CAD build for the part. Positions are in the model's coordinates, mm. A direction names the side the tool comes from. Give positions to 0.01 mm unless a question says otherwise; leave off trailing zeros. Write each loop counter-clockwise with the first axis right and the second up, starting at its lowest first coordinate (ties: lowest second). Pieces come first, ordered by that corner, then holes. Notation, with made-up numbers: (86, -18) - (116, -18) arc R29 cw to (116, 3) - close; hole circle Ø3 at (33, -35). An arc over 180 degrees is marked (long way). Answer as a JSON object with one key per item and string values.
Autodesk Inventor part; units mm, degrees
ref_plane "Work Plane1" through (1.525, 0, 0) normal (0, 0, 1) x (1, 0, 0)
ref_plane "YZ Plane" through (0, 0, 0) normal (1, 0, 0) x (0, 1, 0)
ref_plane "XZ Plane" through (0, 0, 0) normal (0, 1, 0) x (-1, 0, 0)
sketch "Sketch1" plane through (0, 0, 0) normal (0, 0, 1) x (1, 0, 0)
  line L0 (0, 3) -> (12, 3)
  line L1 (12, 3) -> (12, 0)
  line L2 (12, 0) -> (0, 0)
  line L3 (-2.4, 0) -> (14.4, 0)
  line L4 (0, -0.6) -> (0, 3.6)
  line L5 (0, 3) -> (0, 0)
  dimension "d2" = 6
  dimension "d59" = 12
revolve "Body" add sketch "Sketch1" angle 360 about axis through (12, 0, 0) along (-1, 0, 0)
sketch "Sketch2" plane through (0, 0, 0) normal (-1, 0, 0) x (0, 0, 1)
  line L0 (0, 5.7735) -> (5, 2.8868)
  line L1 (5, 2.8868) -> (5, -2.8868)
  line L2 (5, -2.8868) -> (0, -5.7735)
  line L3 (0, -5.7735) -> (-5, -2.8868)
  line L4 (-5, -2.8868) -> (-5, 2.8868)
  line L5 (-5, 2.8868) -> (0, 5.7735)
  line L6 (-7, 0) -> (7, 0)
  line L7 (0, 8.0829) -> (0, -8.0829)
  point P0 (0, 0)
  point P1 (0, 0)
  dimension "d11" = 10
extrude "Head" add sketch "Sketch2" along normal blind 4
sketch "Sketch4" plane through (0, 0, 0) normal (0, 0, 1) x (1, 0, 0)
  line L0 (-3.4226, 6) -> (-4, 5)
  line L1 (-1.1, 0) -> (-0.234, 0)
  line L2 (-4.7532, 0) -> (0.5192, 0)
  line L3 (-4, 6) -> (-3.4226, 6)
  line L4 (-4, 5) -> (-4, 6)
  line L5 (0, 7.2) -> (0, -1.2)
  dimension "d65" = 10
  dimension "d67" = 30
  dimension "d68" = 12
  dimension "d69" = 4
revolve "Chamfer1" cut sketch "Sketch4" angle 360 about axis through (-1.1, 0, 0) along (1, 0, 0)
thread "Thread"
chamfer "Chamfer2" distance 0.6135 distance2 0.6136 1 edges at (12, -3, 0) measured on face at (12, -0.8855, 0.4647)
fillet "Fillet2" radius 0.25 1 edges at (0, -3, 0)
ref_plane "Work Plane1" through (1.525, 0, 0) normal (0, 0, 1) x (1, 0, 0)
equation "\"d2\" = GD"
equation "\"d59\" = NLG"
equation "\"d11\" = SW"
equation "\"d3\" = KOH"
equation "\"d71\" = RR"
equation "\"d15\" = GEL"
equation "\"d6\" = -0.5 * SPD + 0.5 * GD"
equation "\"d65\" = SW"
equation "\"d67\" = ANG1"
equation "\"d68\" = 1.2 * SW"
equation "\"d69\" = KOH"
equation "\"NLG\" = 12"
equation "\"GD\" = NND"
equation "\"BDM\" = NND"
equation "\"KOH\" = 4"
equation "\"GEL\" = 11"
equation "\"SW\" = 10"
equation "\"SPD\" = NND - 1.2269 * PTC"
equation "\"SD2\" = NND"
equation "\"SD\" = 0"
equation "\"ANG1\" = 30deg"
equation "\"GAL\" = 0.61345 * PTC"
equation "\"GUL\" = 0.61345 * PTC"
equation "\"RR\" = 0.25"
equation "\"RR1\" = 0.1"
equation "\"WFT\" = 0"
equation "\"GD1\" = THREADDIA - 1.2269 * PTC"
equation "\"THREADDIA\" = 6"
equation "\"TOA\" = 30deg"
equation "\"FAWI\" = 90deg"
equation "\"PTC\" = 1"
equation "\"NND\" = 6"
equation "\"E0\" = 1.155 * SW"
properties part number "Hexagon bolt GB/T 5781 M6 x 12" material "Steel, Mild"
(1) Flat gauge pins, fed straight in: P1, Ø3, axis at x = 3, z = -2.5, coming from the +Y side; P2, Ø5, axis at x = 2, z = 3.5, coming from the -Y side; P3, Ø4, axis at x = 5.5, y = -1.5, coming from the -Z side. Where does each tip first touch, or does it go through?
Answer key:
{"P1": "stops at y = 2.83", "P2": "stops at y = -4.62", "P3": "stops at z = -3"}
(2) 3-axis set-ups, long thin cutter, end or side, ignore diameter. For faces 1 (the face through (-2, 0, -5)), 2 (the face through (6, -3, 0)): which of +Z, -Z, +X, -X, +Y, -Y reach the whole face in a straight line?
Answer key:
{"face 1": "-Z, +X, -X, +Y, -Y", "face 2": "+X"}
(3) Probe L1, parallel to Z at x = 3.75, y = 0; L2, parallel to X at y = -0.75, z = -3.5; L3, parallel to Y at x = -3, z = 2.75. List the from-to ranges inside material, lowest first. Write a range as [from, to].
Answer key:
{"L1": "z = [-3, 3]", "L2": "x = [-4, 0]", "L3": "y = [-4.19, 4.19]"}
(4) Saw through at A-A, the plane x = -3. Give the cut face in (y, z).
Answer key:
{"outline": "(-5.77, 0) - (-2.89, -5) - (2.89, -5) - (5.77, 0) - (2.89, 5) - (-2.89, 5) - close"}
(5) Saw through at B-B, the plane x = 4. Give the cut face in (y, z).
Answer key:
{"outline": "circle Ø6 at (0, 0)"}
